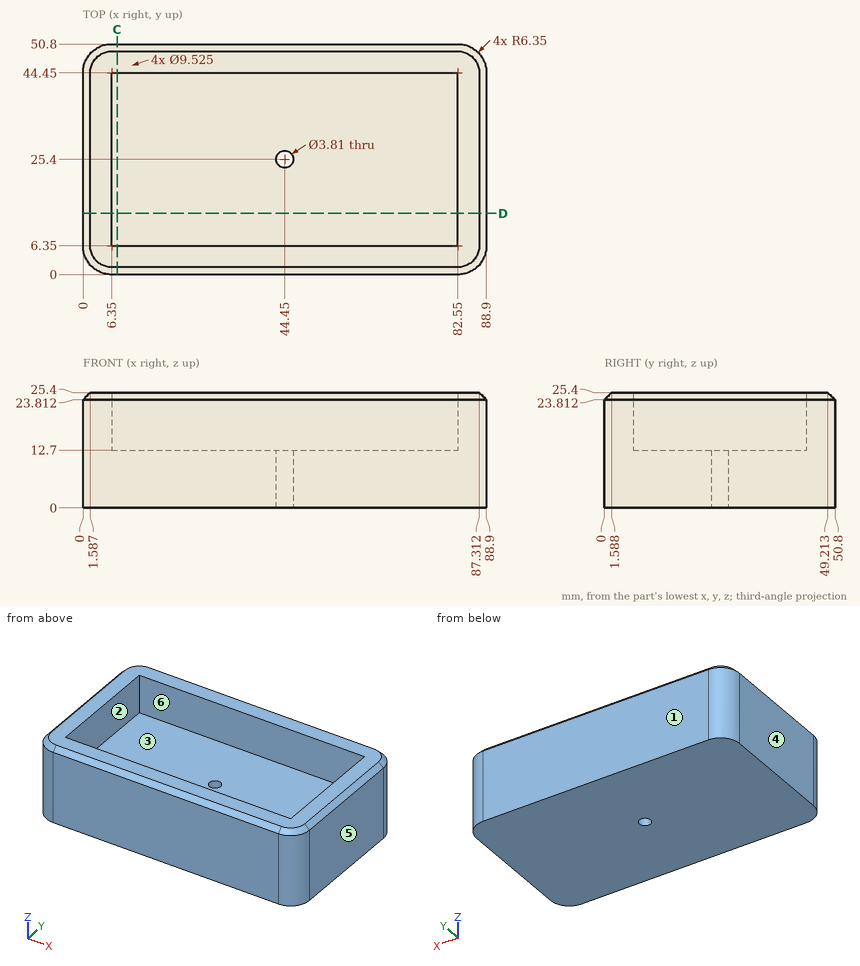
Input: dimensioned drawing with shaded views. Units: mm. Origin: part minimum x, y, z. A direction names the side the tool comes from. Round coordinates to 2 decimals unless told otherwise and drop trailing zeros. Order: outer loops, then holes, each group sorted by start corner. A loop starts at its lowest first (then second) coordinate and runs counter-clockwise, first axis right, second up.
1. Cut plane D-D, the plane y = 13.5. Output: boundary loops of the cut face in (x, z).
The answers:
outline: (0, 0) - (88.9, 0) - (88.9, 23.81) - (87.31, 25.4) - (82.55, 25.4) - (82.55, 12.7) - (6.35, 12.7) - (6.35, 25.4) - (1.59, 25.4) - (0, 23.81) - close
2. Set-up query: the marked faces 5 and 6. Return all of +Z, -Z, +X, -X, +Y, -Y with unobstructed straight access to the full face (end or side cutting, diameter ignored); none if empty.
The answers:
face 5: +Z, -Z, +X, +Y, -Y
face 6: +Z
3. Cut plane C-C, the plane x = 7.5. Output: boundary loops of the cut face in (y, z).
The answers:
outline: (0, 0) - (50.8, 0) - (50.8, 23.81) - (49.21, 25.4) - (44.45, 25.4) - (44.45, 12.7) - (6.35, 12.7) - (6.35, 25.4) - (1.59, 25.4) - (0, 23.81) - close
4. Mould query, pull axis X, two halves, no side actions, for the marked faces 1, 2, 3 and 4. Classes: released by +X, released by -X, zero draft, split by the parting line, or undercut.
The answers:
face 1: zero draft
face 2: undercut
face 3: undercut
face 4: released by -X
5. Pin query (flat end, axial travel): P1, Ø1, axis at x = 43, y = 37, coming from the +Z side; P2, Ø3, axis at x = 44.45, y = 25.4, coming from the -Z side. Return the tip coordinate at first contact, or that it passes through.
The answers:
P1: stops at z = 12.7
P2: passes through
6. Material intervals for line 1 (Y direction, x = 75.5, z = 21.25); line 2 (Y direction, x = 44.45, z = 10) (1 decimal); line 3 (X direction, y = 8.5, z = 16.5), sorted ascending.
The answers:
line 1: y = 0 to 6.35, 44.45 to 50.8
line 2: y = 0 to 23.5, 27.3 to 50.8
line 3: x = 0 to 6.35, 82.55 to 88.9
